Study the drawing (mm; zero at the part's minimum x, y, z) and answer. A direction names the side the tool comes from. Coordinates: 2 decimals unless noted, no trailing zeros. Loops run counter-clockwise (first coordinate to the right, second up) from the corner with the lowest first, then second, coordinate; pieces in that order, holes last. Notation, with made-up numbers: (18, -20.5) - (32, -20.5) arc R17 cw to (32, -8.5) - close; hole circle Ø6 at (51.5, 9.5). An arc over 180 degrees is marked (long way). Write each question's results on one line, items separated by ' | '. Start each with the question number.
(1) For the marked faces 1, 2 and 3, determine the directions among +Z, -Z, +X, -X, +Y, -Y from which every point of the face is accessible in a straight line to the end or side of a thin tool.
(2) Find section A-A on z = 57. Determine the outline of the cut face in (x, y).
(3) Given pin 1 Ø8 at (y, z) = (66.5, 33) entering from -X; pin 2 Ø23 at (x, y) = (50.5, 33.5) entering from -Z; pin 3 Ø4 at (y, z) = (70, 18.5) entering from -X; pin 4 Ø4 at (x, z) = (38.1, 12.7) entering from -Y, each flat-ended and moving along its own axis, determine where each tip first touches the part or whether it passes through.
(4) Find section B-B on x = 38.1. Determine the outline of the cut face in (y, z) (3 decimals).
(5) Determine the mould class of the marked faces 4, 5, 6 and 7 for opening direction X: released by +X, released by -X, zero draft, split by the parting line, or undercut.
(6) Consider line 1 (Z direction, x = 5.75, y = 38.1) (3 decimals); line 2 (X direction, y = 50, z = 61.5); line 3 (Z direction, x = 38, y = 6). Determine where each line is inside the solid, lowest interval first. Write a range as from..to.
(7) Find section D-D on z = 28. Determine the outline of the cut face in (x, y).
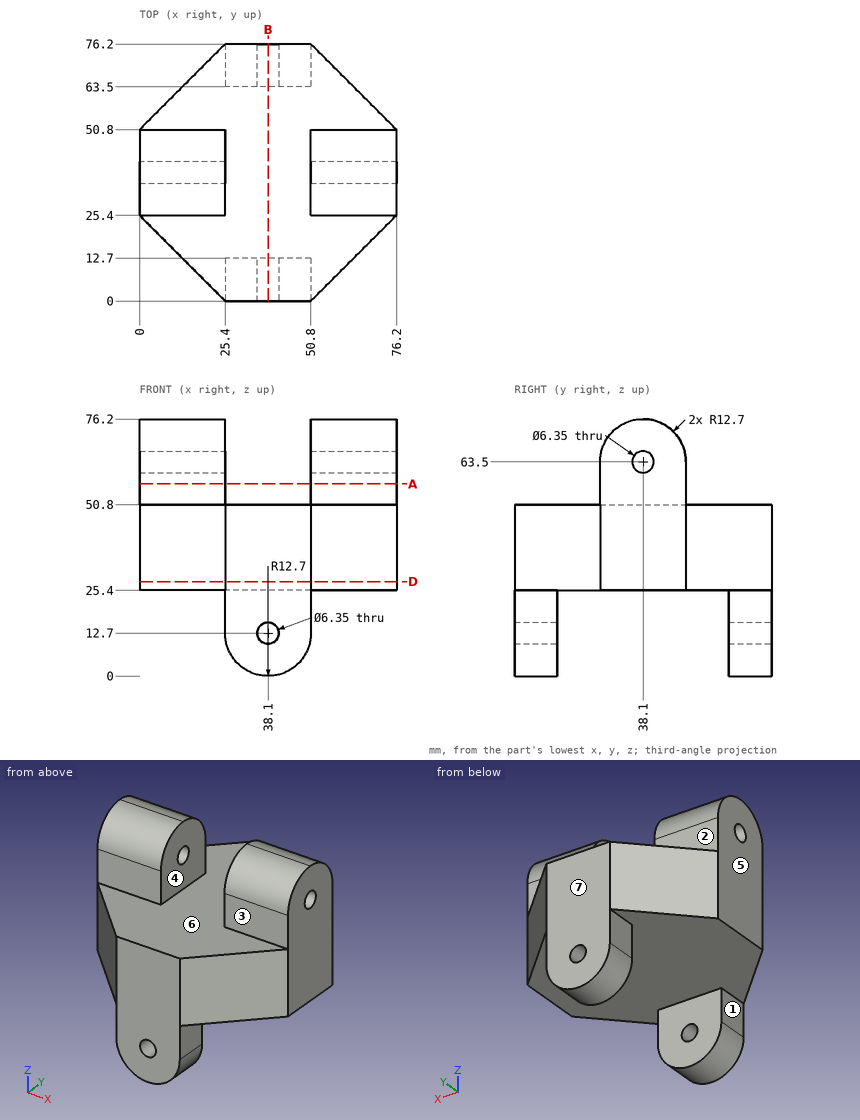
Values:
1) face 1: -Z, -X, +Y, -Y | face 2: +Z, +X, -X, +Y | face 3: +Z, +X, -X, -Y
2) outline: (0, 25.4) - (25.4, 25.4) - (25.4, 50.8) - (0, 50.8) - close; (50.8, 25.4) - (76.2, 25.4) - (76.2, 50.8) - (50.8, 50.8) - close
3) pin 1: stops at x = 11.7 | pin 2: stops at z = 25.4 | pin 3: stops at x = 25.4 | pin 4: passes through
4) outline: (0, 0) - (12.7, 0) - (12.7, 9.525) - (0, 9.525) - close; (0, 15.875) - (12.7, 15.875) - (12.7, 25.4) - (63.5, 25.4) - (63.5, 15.875) - (76.2, 15.875) - (76.2, 50.8) - (0, 50.8) - close; (63.5, 0) - (76.2, 0) - (76.2, 9.525) - (63.5, 9.525) - close
5) face 4: undercut | face 5: released by -X | face 6: undercut | face 7: zero draft
6) line 1: z = 25.4..60.325, 66.675..76.2 | line 2: x = 0..25.4, 50.8..76.2 | line 3: z = 0..9.53, 15.87..50.8
7) outline: (0, 25.4) - (25.4, 0) - (50.8, 0) - (76.2, 25.4) - (76.2, 50.8) - (50.8, 76.2) - (25.4, 76.2) - (0, 50.8) - close
